from build123d import *

# Parameters (mm, degrees)
SKETCH1_R           = 3.2385
BOSS_EXTRUDE1_DEPTH = 12.7
SKETCH2_R           = 6.35
SKETCH2_W           = 44.45
SKETCH2_H           = 19.05
CUT_EXTRUDE1_DEPTH  = 6.35
BOSS_EXTRUDE4_DEPTH = 12.7
FILLET1_R           = 20
SKETCH4_R           = 3.2385
BOSS_EXTRUDE5_DEPTH = 12.7
SKETCH5_W           = 25.4
SKETCH5_H           = 19.05
CUT_EXTRUDE2_DEPTH  = 6.35


with BuildPart() as part:
    # Sketch1 → Boss-Extrude1 (new body)
    with BuildSketch(Plane(origin=(0, 0, 0), x_dir=(1, 0, 0), z_dir=(0, 1, 0))):
        Polygon((0, 0), (-39.00058596, 101.6), (-39.00058596, 120.65), (5.44941404, 120.65), (5.44941404, 101.6), (44.45, 0), align=None)
        with Locations((17.673727041, 11.856471417)):
            Circle(SKETCH1_R, mode=Mode.SUBTRACT)
        with Locations((-16.77558596, 111.125)):
            Circle(SKETCH1_R, mode=Mode.SUBTRACT)
    extrude(amount=BOSS_EXTRUDE1_DEPTH)

    # Sketch2 → Cut-Extrude1 (cut)
    with BuildSketch(Plane(origin=(0, 12.7, 0), x_dir=(1, 0, 0), z_dir=(0, 1, 0))):
        with Locations((17.673727041, 11.856471417)):
            Circle(SKETCH2_R)
        with Locations((-16.77558596, 111.125)):
            Rectangle(SKETCH2_W, SKETCH2_H)
    extrude(amount=-CUT_EXTRUDE1_DEPTH, mode=Mode.SUBTRACT)

    # Sketch3 → Boss-Extrude4 (add)
    with BuildSketch(Plane(origin=(0, 12.7, 0), x_dir=(1, 0, 0), z_dir=(0, 1, 0))):
        with BuildLine():
            Line((32.408197765, 120.65), (5.44941404, 120.65))
            Line((5.44941404, 120.65), (5.44941404, 104.775))
            ThreePointArc((5.44941404, 104.775), (4.519478071, 102.52993597), (2.27441404, 101.6))
            Line((2.27441404, 101.6), (5.44941404, 101.6))
            ThreePointArc((5.44941404, 101.6), (16.992497649, 113.865184538), (32.408197765, 120.65))
        make_face()
    extrude(amount=-BOSS_EXTRUDE4_DEPTH)

    # Fillet1
    fillet1_edges = [part.edges().sort_by_distance(p)[0] for p in [
        (5.44941404, 6.35, -101.6),
    ]]
    fillet(fillet1_edges, radius=FILLET1_R)

    # Sketch4 → Boss-Extrude5 (add)
    with BuildSketch(Plane(origin=(0, 0, 0), x_dir=(1, 0, 0), z_dir=(0, 1, 0))):
        with BuildLine():
            Line((-80.27558596, 101.926821939), (-80.27558596, 90.176821939))
            ThreePointArc((-80.27558596, 90.176821939), (-74.417721583, 76.034686315), (-60.27558596, 70.176821939))
            Line((-60.27558596, 70.176821939), (-26.938358036, 70.176821939))
            Line((-26.938358036, 70.176821939), (-25.01903786, 65.176821939))
            Line((-25.01903786, 65.176821939), (-60.27558596, 65.176821939))
            ThreePointArc((-60.27558596, 65.176821939), (-76.539652165, 71.190507118), (-84.979160459, 86.338409901))
            ThreePointArc((-84.979160459, 86.338409901), (-92.17483168, 98.279259247), (-105.67558596, 101.75649972))
            Line((-105.67558596, 101.75649972), (-105.67558596, 120.80649972))
            Line((-105.67558596, 120.80649972), (-80.27558596, 120.80649972))
            Line((-80.27558596, 120.80649972), (-80.27558596, 101.926821939))
        make_face()
        with Locations((-92.97558596, 111.36666083)):
            Circle(SKETCH4_R, mode=Mode.SUBTRACT)
    extrude(amount=BOSS_EXTRUDE5_DEPTH)

    # Sketch5 → Cut-Extrude2 (cut)
    with BuildSketch(Plane(origin=(0, 12.7, 0), x_dir=(1, 0, 0), z_dir=(0, 1, 0))):
        with Locations((-92.97558596, 111.28149972)):
            Rectangle(SKETCH5_W, SKETCH5_H)
    extrude(amount=-CUT_EXTRUDE2_DEPTH, mode=Mode.SUBTRACT)


solid = part.part
Here's how the part is built. I have some questions about the finished solid (model axes, mm). A direction names the side the tool comes from. Coordinates: 2 decimals unless noted, no trailing zeros. Write each loop counter-clockwise with the first axis right and the second up, starting at its lowest first coordinate (ties: lowest second). Pieces come first, ordered by that corner, then holes.
1) If we section it at A-A (x = -37): List the corners of the cut face in (y, z) for me.
Filled in:
outline: (0, -120.65) - (6.35, -120.65) - (6.35, -101.6) - (12.7, -101.6) - (12.7, -96.39) - (0, -96.39) - close; (0, -70.18) - (12.7, -70.18) - (12.7, -65.18) - (0, -65.18) - close
2) If we section it at C-C (y = 3.5): Count the separate pieces of the cut face and the enclosed holes in it, plus the area to 3 significant figures.
Filled in:
separate pieces: 1
enclosed holes: 3
area: 6,430 mm2
3) Thinking about a two-plate mould opening in Z: for faces 1 (the face through (-91, 10, -101.756)), 2 (the face through (20.6, 9.57, -6.22)), 3 (the face through (-15, 0, -75)), 4 (the face through (-42, 6, -65.177)), which applies, +Z half, -Z half, draft (parallel to the pull), parting line (faces both ways), or undercut?
Filled in:
face 1: -Z half
face 2: undercut
face 3: draft
face 4: +Z half
4) I'm going to push flat-ended pins straight in: pin 1 (15 mm diameter, centred on x = -97, z = -113.5, fed in from +Y); pin 2 (6.5 mm diameter, centred on x = -36, y = 6.5, fed in from +Z); pin 3 (3 mm diameter, centred on y = 10, z = -15, fed in from -X). Where does each tip first touch, or does it pass through?
Filled in:
pin 1: stops at y = 6.35
pin 2: stops at z = -65.18
pin 3: stops at x = -6.33
5) If we section it at D-D (x = -82.5): List the corners of the cut face in (y, z) for me, plus the area to 3 significant figures.
Filled in:
outline: (0, -120.81) - (6.35, -120.81) - (6.35, -101.76) - (12.7, -101.76) - (12.7, -78.73) - (0, -78.73) - close
area: 413 mm2
6) If we section it at B-B (z = -77): List the corners of the cut face in (x, y) for me.
Filled in:
outline: (-81.52, 0) - (-75.32, 0) - (-75.32, 12.7) - (-81.52, 12.7) - close; (-29.56, 0) - (14.89, 0) - (14.89, 12.7) - (-29.56, 12.7) - close
7) If I drill on line 1 (X direction, y = 10, z = -88); line 2 (Z direction, x = -56.5, y = 1); line 3 (X direction, y = 3.25, z = -86), over which ranges is the centre line in solid material (lowest first)?
Filled in:
line 1: x = -85.32 to -80.16, -33.78 to 10.67
line 2: z = -70.18 to -65.18
line 3: x = -84.92 to -79.83, -33.01 to 11.44
8) Which directions (+Z, -Z, +X, -X, +Y, -Y) give clear straight access to the entire face, cutting with the end or side of a thin tool? Please do faces 5 (the face through (-80.276, 5, -102)), 6 (the face through (26.874, 6.261, -45.786)), 7 (the face through (4.54, 9.57, -102.55)).
Filled in:
face 5: -Z, +Y, -Y
face 6: +X, +Y, -Y
face 7: -Z, +Y
